Input: part model. Units: mm. Frame: model coordinates. Face numbers are marked on the shaded views. Coordinates: 2 decimals unless noted, no trailing zeros. Order: outer loops, then holes, each group sorted by start corner. A loop starts at its lowest first (then second) coordinate and runs counter-clockwise, first axis right, second up. Notation, with made-up numbers: M 40.5,23.5 L 91.5,23.5 A20 cw 91.5,56.5 Z; hole C 59,76 d10. An arc over 180 degrees is marked long. One line per item, written item: value.
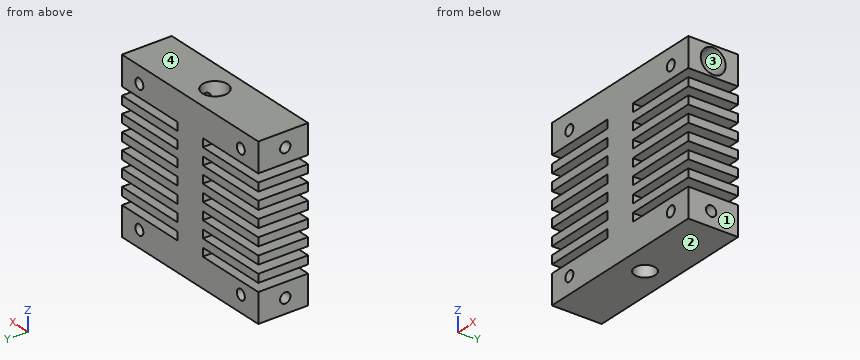
```python
from build123d import *

# Parameters (mm, degrees)
SKETCH_1_W              = 43
SKETCH_1_H              = 40
EXTRUDE_1_DEPTH         = 2
SKETCH_3_W              = 43
SKETCH_3_H              = 40
EXTRUDE_3_DEPTH         = 10
SKETCH_4_R              = 3.025
CUT_EXTRUDE_1_DEPTH     = 20
CUT_EXTRUDE_2_REACH     = 48.971
SKETCH_5_R              = 2.025
HOLE_WIZARD_M6_1_D      = 5
HOLE_WIZARD_M6_1_DEPTH  = 8
SKETCH_8_W              = 17.5
SKETCH_8_H              = 2
CUT_EXTRUDE_3_DEPTH     = 12
HOLE_WIZARD_M3_1_D      = 2.5
HOLE_WIZARD_M3_2_D      = 2.5
HOLE_WIZARD_M3_2_DEPTH  = 4
HOLE_WIZARD_M3_3_D      = 2.5
HOLE_WIZARD_M3_3_DEPTH  = 4
SKETCH_16_R             = 3
CUT_EXTRUDE_4_DEPTH     = 13.5
HOLE_WIZARD_M3_4_REACH  = 39.607
HOLE_WIZARD_M3_4_BORE_R = 1.25


with BuildPart() as part:
    # 草图1 → 凸台-拉伸1 (new body)
    with BuildSketch(Plane(origin=(0, 0, 0), x_dir=(1, 0, 0), z_dir=(0, 1, 0))):
        Rectangle(SKETCH_1_W, SKETCH_1_H)
    extrude(amount=EXTRUDE_1_DEPTH)

    # 草图3 → 凸台-拉伸3 (add)
    with BuildSketch(Plane(origin=(0, 2, 0), x_dir=(1, 0, 0), z_dir=(0, 1, 0))):
        Rectangle(SKETCH_3_W, SKETCH_3_H)
    extrude(amount=EXTRUDE_3_DEPTH)

    # 草图4 → 切除-拉伸1 (cut)
    with BuildSketch(Plane.XY.offset(20)):
        with Locations((0, 6)):
            Circle(SKETCH_4_R)
    extrude(amount=-CUT_EXTRUDE_1_DEPTH, mode=Mode.SUBTRACT)

    # 草图5 → 切除-拉伸2 (cut, up to next)
    with BuildSketch(Plane(origin=(0, 0, -20), x_dir=(-1, 0, 0), z_dir=(0, 0, -1)), mode=Mode.PRIVATE) as cut_extrude_2_sk1:
        with Locations((0, 6)):
            Circle(SKETCH_5_R)
    cut_extrude_2_tool1 = extrude(cut_extrude_2_sk1.sketch, amount=-CUT_EXTRUDE_2_REACH, mode=Mode.PRIVATE) & part.part
    add(cut_extrude_2_tool1.solids().sort_by_distance((0, 6, -20))[0], mode=Mode.SUBTRACT)

    # M6 螺纹孔1
    with Locations(Plane(origin=(0, 0, -20), x_dir=(-1, 0, 0), z_dir=(0, 0, -1))):
        with Locations((0, 6)):
            Hole(HOLE_WIZARD_M6_1_D / 2, depth=HOLE_WIZARD_M6_1_DEPTH)

    # 草图8 → 切除-拉伸3 (cut)
    with BuildSketch(Plane(origin=(0, 12, 0), x_dir=(1, 0, 0), z_dir=(0, 1, 0))):
        with Locations((-12.75, -12)):
            Rectangle(SKETCH_8_W, SKETCH_8_H)
        with Locations((-12.75, -8)):
            Rectangle(SKETCH_8_W, SKETCH_8_H)
        with Locations((-12.75, -4)):
            Rectangle(SKETCH_8_W, SKETCH_8_H)
        with Locations((-12.75, 0)):
            Rectangle(SKETCH_8_W, SKETCH_8_H)
        with Locations((-12.75, 4)):
            Rectangle(SKETCH_8_W, SKETCH_8_H)
        with Locations((-12.75, 8)):
            Rectangle(SKETCH_8_W, SKETCH_8_H)
        with Locations((-12.75, 12)):
            Rectangle(SKETCH_8_W, SKETCH_8_H)
        with Locations((12.75, 12)):
            Rectangle(SKETCH_8_W, SKETCH_8_H)
        with Locations((12.75, 8)):
            Rectangle(SKETCH_8_W, SKETCH_8_H)
        with Locations((12.75, 4)):
            Rectangle(SKETCH_8_W, SKETCH_8_H)
        with Locations((12.75, 0)):
            Rectangle(SKETCH_8_W, SKETCH_8_H)
        with Locations((12.75, -4)):
            Rectangle(SKETCH_8_W, SKETCH_8_H)
        with Locations((12.75, -8)):
            Rectangle(SKETCH_8_W, SKETCH_8_H)
        with Locations((12.75, -12)):
            Rectangle(SKETCH_8_W, SKETCH_8_H)
    extrude(amount=-CUT_EXTRUDE_3_DEPTH, mode=Mode.SUBTRACT)

    # M3 螺纹孔1 (through all)
    with Locations(Plane(origin=(0, 12, 0), x_dir=(1, 0, 0), z_dir=(0, 1, 0))):
        with Locations((-16, 16), (16, 16), (-16, -16), (16, -16)):
            Hole(HOLE_WIZARD_M3_1_D / 2)

    # M3 螺纹孔2
    with Locations(Plane(origin=(21.5, 0, 0), x_dir=(0, 0, -1), z_dir=(1, 0, 0))):
        with Locations((16.5, 5.5)):
            Hole(HOLE_WIZARD_M3_2_D / 2, depth=HOLE_WIZARD_M3_2_DEPTH)

    # M3 螺纹孔3
    with Locations(Plane.ZY.offset(21.5)):
        with Locations((-16.5, 5.5), (16.5, 5.5)):
            Hole(HOLE_WIZARD_M3_3_D / 2, depth=HOLE_WIZARD_M3_3_DEPTH)

    # 草图16 → 切除-拉伸4 (cut)
    with BuildSketch(Plane(origin=(21.5, 0, 0), x_dir=(0, 0, -1), z_dir=(1, 0, 0))):
        with Locations((-16.5, 6)):
            Circle(SKETCH_16_R)
    extrude(amount=-CUT_EXTRUDE_4_DEPTH, mode=Mode.SUBTRACT)

    # M3 螺纹孔4 bore → M3 螺纹孔4 (cut, up to next)
    with BuildSketch(Plane(origin=(8, 0, 0), x_dir=(0, 0, -1), z_dir=(1, 0, 0)), mode=Mode.PRIVATE) as hole_wizard_m3_4_sk1:
        with Locations((-16.5, 6)):
            Circle(HOLE_WIZARD_M3_4_BORE_R)
    hole_wizard_m3_4_tool1 = extrude(hole_wizard_m3_4_sk1.sketch, amount=-HOLE_WIZARD_M3_4_REACH, mode=Mode.PRIVATE) & part.part
    add(hole_wizard_m3_4_tool1.solids().sort_by_distance((8, 6, 16.5))[0], mode=Mode.SUBTRACT)


solid = part.part
```
(1) First-contact query: pin 1 (0.6 mm diameter, centred on y = 6, z = -0.5, fed in from +X); pin 2 (6 mm diameter, centred on x = -8.5, z = 2, fed in from -Y); pin 3 (4.5 mm diameter, centred on x = 0, y = 6, fed in from -Z). Flat tips, straight axial feed; report the tip coordinate or a pass-through.
Data:
pin 1: stops at x = 4
pin 2: stops at y = 0
pin 3: stops at z = -12
(2) Cut plane D-D on x = 0. Output: boundary loops of the cut face in (y, z) (3 decimals).
Data:
outline: M 0,-20 L 3.5,-20 L 3.5,-12 L 3.975,-12 L 3.975,0 L 2.975,0 L 2.975,20 L 0,20 Z; M 8.025,-12 L 8.5,-12 L 8.5,-20 L 12,-20 L 12,20 L 9.025,20 L 9.025,0 L 8.025,0 Z
(3) Draft query along Z for the marked faces 1, 2, 3 and 4. Return one class per face: released by +Z, released by -Z, zero draft, split by the parting line, or undercut.
Data:
face 1: zero draft
face 2: released by -Z
face 3: undercut
face 4: released by +Z
(4) Cut plane A-A on x = -18. Give the number of separate pieces and of enclosed holes in the cut face, plus the area to 3 significant figures.
Data:
separate pieces: 8
enclosed holes: 2
area: 302 mm2
(5) Cut plane C-C on z = -16. Output: boundary loops of the cut face in (x, y).
Data:
outline: M -21.5,0 L -17.25,0 L -17.25,12 L -21.5,12 L -21.5,6.65 L -17.5,6.65 L -17.5,4.35 L -21.5,4.35 Z; M -14.75,0 L 14.75,0 L 14.75,12 L -14.75,12 Z; M 17.25,0 L 21.5,0 L 21.5,4.35 L 17.5,4.35 L 17.5,6.65 L 21.5,6.65 L 21.5,12 L 17.25,12 Z; hole C 0,6 d5
(6) Ray query, line 1 (X direction, y = 9, z = -16); line 2 (Y direction, x = -19.5, z = -16.5); line 3 (X direction, y = 11, z = 15). Return the intervals inside material, ascending. Write a range as from..to.
Data:
line 1: x = -21.5..-17.25, -14.75..14.75, 17.25..21.5
line 2: y = 0..4.25, 6.75..12
line 3: x = -21.5..-16.75, -15.25..15.25, 16.75..21.5
